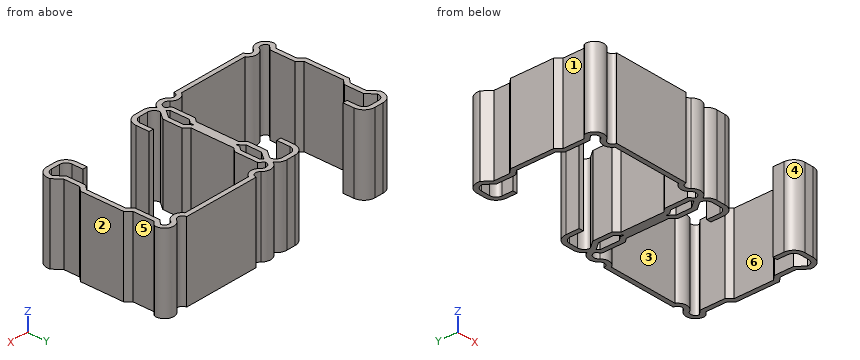
```python
from build123d import *

# Parameters (mm, degrees)
BASE_EXTRUDE_DEPTH = 12.7
CIRPATTERN1_COUNT  = 2


with BuildPart() as part:
    # Sketch1 → Base-Extrude (new, symmetric)
    with BuildSketch(Plane(origin=(-20.32, 17.78, 0), x_dir=(1, 0, 0), z_dir=(0, 0, 1))):
        with BuildLine():
            Line((17.3228, 17.075886512), (19.412382578, 19.800133504))
            ThreePointArc((19.412382578, 19.800133504), (18.838545845, 21.346344632), (17.3228, 21.9964))
            Line((17.3228, 21.9964), (14.38577367, 21.9964))
            ThreePointArc((14.38577367, 21.9964), (12.906383481, 21.383616519), (12.2936, 19.90422633))
            Line((12.2936, 19.90422633), (12.2936, 15.61465))
            Line((12.2936, 15.61465), (10.795, 15.61465))
            Line((10.795, 15.61465), (10.795, 19.90422633))
            ThreePointArc((10.795, 19.90422633), (11.846713258, 22.443286742), (14.38577367, 23.495))
            Line((14.38577367, 23.495), (17.3228, 23.495))
            ThreePointArc((17.3228, 23.495), (20.097934554, 22.182884653), (20.844928673, 19.2054666))
            Line((20.844928673, 19.2054666), (18.8214, 16.567335923))
            Line((18.8214, 16.567335923), (18.8214, 11.485729415))
            Line((18.8214, 11.485729415), (20.32, 9.8028125))
            Line((20.32, 9.8028125), (20.32, -5.180962694))
            Line((20.32, -5.180962694), (19.1389, -6.507329415))
            Line((19.1389, -6.507329415), (19.1389, -12.757931546))
            Line((19.1389, -12.757931546), (20.424084837, -14.043116383))
            ThreePointArc((20.424084837, -14.043116383), (18.821804006, -17.54486751), (15.019825564, -16.932883251))
            ThreePointArc((15.019825564, -16.932883251), (13.348875824, -16.363652979), (12.29528328, -17.78))
            Line((12.29528328, -17.78), (-12.61278328, -17.78))
            ThreePointArc((-12.61278328, -17.78), (-13.666375824, -16.363652979), (-15.337325564, -16.932883251))
            ThreePointArc((-15.337325564, -16.932883251), (-19.047442105, -18.270236732), (-20.870958003, -14.773342558))
            Line((-20.870958003, -14.773342558), (-19.4564, -13.358784555))
            Line((-19.4564, -13.358784555), (-19.4564, -6.507329415))
            Line((-19.4564, -6.507329415), (-20.955, -4.8244125))
            Line((-20.955, -4.8244125), (-20.955, 9.0662125))
            Line((-20.955, 9.0662125), (-19.4564, 10.749129415))
            Line((-19.4564, 10.749129415), (-19.4564, 15.830735923))
            Line((-19.4564, 15.830735923), (-21.479928673, 18.4688666))
            ThreePointArc((-21.479928673, 18.4688666), (-20.732934554, 21.446284653), (-17.9578, 22.7584))
            Line((-17.9578, 22.7584), (-15.02077367, 22.7584))
            ThreePointArc((-15.02077367, 22.7584), (-12.481713258, 21.706686742), (-11.43, 19.16762633))
            Line((-11.43, 19.16762633), (-11.43, 15.61465))
            Line((-11.43, 15.61465), (-12.9286, 15.61465))
            Line((-12.9286, 15.61465), (-12.9286, 19.16762633))
            ThreePointArc((-12.9286, 19.16762633), (-13.541383481, 20.647016519), (-15.02077367, 21.2598))
            Line((-15.02077367, 21.2598), (-17.9578, 21.2598))
            ThreePointArc((-17.9578, 21.2598), (-19.473545845, 20.609744632), (-20.047382578, 19.063533504))
            Line((-20.047382578, 19.063533504), (-17.9578, 16.339286512))
            Line((-17.9578, 16.339286512), (-17.9578, 10.17860201))
            Line((-17.9578, 10.17860201), (-19.4564, 8.495685095))
            Line((-19.4564, 8.495685095), (-19.4564, -4.253885095))
            Line((-19.4564, -4.253885095), (-17.9578, -5.93680201))
            Line((-17.9578, -5.93680201), (-17.9578, -13.979525))
            Line((-17.9578, -13.979525), (-19.4564, -15.478125))
            ThreePointArc((-19.4564, -15.478125), (-18.409738669, -16.906954381), (-16.731785827, -16.33992034))
            ThreePointArc((-16.731785827, -16.33992034), (-14.14499029, -14.797667818), (-11.524190259, -16.2814))
            Line((-11.524190259, -16.2814), (11.206690259, -16.2814))
            ThreePointArc((11.206690259, -16.2814), (13.441553644, -14.818250812), (15.956217628, -15.719297395))
            ThreePointArc((15.956217628, -15.719297395), (17.836242029, -16.3415136), (19.00315301, -14.741525))
            Line((19.00315301, -14.741525), (17.6403, -13.37867199))
            Line((17.6403, -13.37867199), (17.6403, -5.93680201))
            Line((17.6403, -5.93680201), (18.8214, -4.610435289))
            Line((18.8214, -4.610435289), (18.8214, 9.232285095))
            Line((18.8214, 9.232285095), (17.3228, 10.91520201))
            Line((17.3228, 10.91520201), (17.3228, 17.075886512))
        make_face()
    base_extrude = extrude(amount=BASE_EXTRUDE_DEPTH, both=True)

    # CirPattern1: Base-Extrude ×2 about axis
    cirpattern1_axis = Axis((0, 20.6375, 0), (0, 0, 1))
    for i in range(1, CIRPATTERN1_COUNT):
        add(base_extrude.rotate(cirpattern1_axis, i * 360 / CIRPATTERN1_COUNT))


solid = part.part
```
Read the model definition and answer for the solid it produces. Units are mm, in the model's axes. Face numbers are marked on the shaded views. A direction names the side the tool comes from. Give positions to 0.01 mm unless a question says otherwise; leave off trailing zeros. Order: outer loops, then holes, each group sorted by start corner. A loop starts at its lowest first (then second) coordinate and runs counter-clockwise, first axis right, second up.
(1) Find section A-A (y = 32). Give the vertices of the cut face in (x, z), plus the area to 3 significant figures.
(2) Straight lines are drawn through the part: L1, parallel to X at y = 21.5, z = 9.5 (3 decimals); L2, parallel to X at y = 8, z = 2; L3, parallel to X at y = 7.5, z = 11.25 (3 decimals). For each, find the intervals that lie inside material, in ascending order.
(3) Find section C-C (z = 11). Give the number of separate pieces and of enclosed holes in the cut face, plus the area to 3 significant figures.
(4) Find section B-B (x = -22). Give the vertices of the cut face in (y, z), plus the area to 3 significant figures.
(5) Given pin 1 (12 mm diameter, centred on y = 30.5, z = 2.5, fed in from -X); pin 2 (1.1 mm diameter, centred on y = 36, z = 5.5, fed in from +X); pin 3 (0.9 mm diameter, centred on x = -37, z = 4.5, fed in from -Y), each flat-ended and moving along its own axis, determine where each tip first touches the part or whether it passes through.
(6) For the marked faces 4, 5 and 6, determine the directions among +Z, -Z, +X, -X, +Y, -Y from which every point of the face is accessible in a straight line to the end or side of a thin tool.
(7) For a pull along X with two mould halves and no side action, classify the marked faces 1, 2 and 3 as released by +X, released by -X, zero draft, split by the parting line, or undercut.
Result sheet:
1. outline: (-39.78, -12.7) - (-38.28, -12.7) - (-38.28, 12.7) - (-39.78, 12.7) - close; (-3, -12.7) - (-1.5, -12.7) - (-1.5, 12.7) - (-3, 12.7) - close; (1.18, -12.7) - (2.68, -12.7) - (2.68, 12.7) - (1.18, 12.7) - close; (38.28, -12.7) - (39.78, -12.7) - (39.78, 12.7) - (38.28, 12.7) - close
1. area: 152 mm2
2. L1: x = -41.275 to -39.776, -1.499 to 1.499, 39.776 to 41.275
2. L2: x = -39.78 to -38.28, -2.68 to -1.18, 1.5 to 3, 38.28 to 39.78
2. L3: x = -39.776 to -38.278, -2.68 to -1.181, 1.499 to 2.997, 8.026 to 9.525, 31.75 to 33.249, 38.278 to 39.902
3. separate pieces: 1
3. enclosed holes: 2
3. area: 449 mm2
4. outline: (0, -12.7) - (1.5, -12.7) - (1.5, 12.7) - (0, 12.7) - close
4. area: 38.1 mm2
5. pin 1: stops at x = -41.84
5. pin 2: stops at x = 39.78
5. pin 3: stops at y = -0.58
6. face 4: +Z, -Z, -Y
6. face 5: +Z, -Z, +X
6. face 6: +Z, -Z
7. face 1: released by -X
7. face 2: released by +X
7. face 3: undercut
